Geometry check sheet. Reference: drawing and pictorial views, mm from the part's lowest x, y, z. A direction names the side the tool comes from. Give positions to 0.01 mm unless a question says otherwise; leave off trailing zeros. Write each loop counter-clockwise with the first axis right and the second up, starting at its lowest first coordinate (ties: lowest second). Pieces come first, ordered by that corner, then holes.
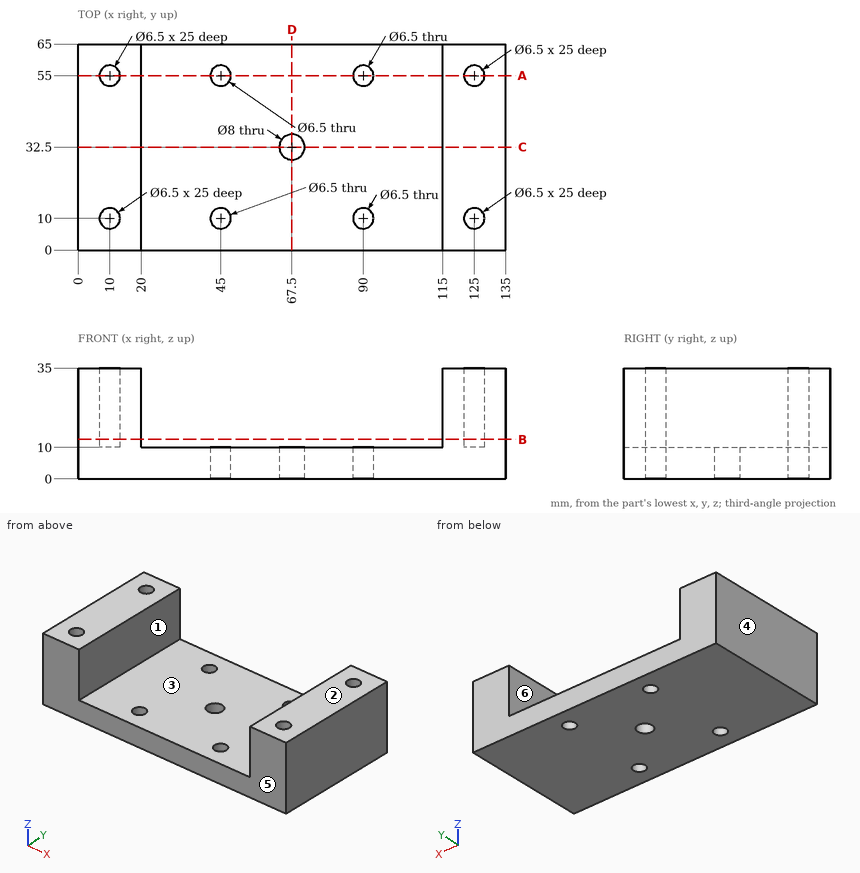
Item 1: Set-up check for the marked faces 5 and 6: record each of +Z, -Z, +X, -X, +Y, -Y from which the full face is reachable in a straight line by a thin tool's end or side.
Answer key:
face 5: +Z, -Z, +X, -X, -Y
face 6: +Z, +Y, -Y
Item 2: Sectioned sample at A-A on y = 55. Record the cut outline in (x, z), then the cut area to 4 significant figures.
Answer key:
outline: (0, 0) - (41.75, 0) - (41.75, 10) - (20, 10) - (20, 35) - (13.25, 35) - (13.25, 10) - (6.75, 10) - (6.75, 35) - (0, 35) - close; (48.25, 0) - (86.75, 0) - (86.75, 10) - (48.25, 10) - close; (93.25, 0) - (135, 0) - (135, 35) - (128.25, 35) - (128.25, 10) - (121.75, 10) - (121.75, 35) - (115, 35) - (115, 10) - (93.25, 10) - close
area: 1,895 mm2
Item 3: Release check for a two-part mould opening along X. For the marked faces 1, 2, 3 and 4 record: released by +X, released by -X, zero draft, split by the parting line, or undercut.
Answer key:
face 1: undercut
face 2: zero draft
face 3: undercut
face 4: released by -X
Item 4: Sectioned sample at D-D on x = 67.5. Record the cut outline in (y, z), then the cut area to 3 significant figures.
Answer key:
outline: (0, 0) - (28.5, 0) - (28.5, 10) - (0, 10) - close; (36.5, 0) - (65, 0) - (65, 10) - (36.5, 10) - close
area: 570 mm2
Item 5: Scan lines: line 1 along Y through (x, z) = (90, 5.75); line 2 along X through (y, z) = (23.5, 32); line 3 along Y through (x, z) = (93, 5.5). Record each from-to range of solid material in increasing order.
Answer key:
line 1: y = 0 to 6.75, 13.25 to 51.75, 58.25 to 65
line 2: x = 0 to 20, 115 to 135
line 3: y = 0 to 8.75, 11.25 to 53.75, 56.25 to 65
Item 6: Sectioned sample at C-C on y = 32.5. Record the cut outline in (x, z), then the cut area to 3 significant figures.
Answer key:
outline: (0, 0) - (63.5, 0) - (63.5, 10) - (20, 10) - (20, 35) - (0, 35) - close; (71.5, 0) - (135, 0) - (135, 35) - (115, 35) - (115, 10) - (71.5, 10) - close
area: 2,270 mm2
Item 7: Depth check by flat-ended pin: pin 1 (19.5 mm diameter, centred on x = 58, y = 29, fed in from +Z). Enter the tip coordinate at first touch or a pass-through.
Answer key:
pin 1: stops at z = 10
Item 8: Sectioned sample at B-B on z = 12.5. Record the cut outline in (x, y), then the cut area to 3 significant figures.
Answer key:
outline: (0, 0) - (20, 0) - (20, 65) - (0, 65) - close; (115, 0) - (135, 0) - (135, 65) - (115, 65) - close; hole circle Ø6.5 at (10, 10); hole circle Ø6.5 at (10, 55); hole circle Ø6.5 at (125, 10); hole circle Ø6.5 at (125, 55)
area: 2,470 mm2
